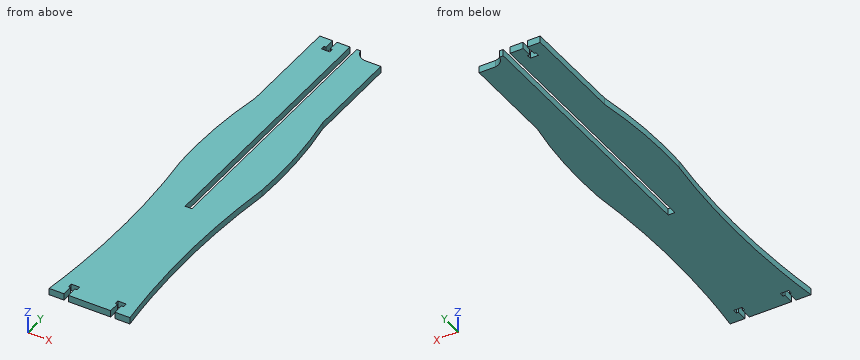
from build123d import *

# Parameters (mm, degrees)
BOSS_EXTRUDE1_DEPTH = 6.35


with BuildPart() as part:
    # Sketch2 → Boss-Extrude1 (new body)
    with BuildSketch(Plane.XY):
        with BuildLine():
            Line((-41.275, 0), (-27.223297828, 0))
            Line((-27.223297828, 0), (-27.223297828, 10.16))
            Line((-27.223297828, 10.16), (-29.128297828, 10.16))
            Line((-29.128297828, 10.16), (-29.128297828, 14.224))
            Line((-29.128297828, 14.224), (-21.254297828, 14.224))
            Line((-21.254297828, 14.224), (-21.254297828, 10.16))
            Line((-21.254297828, 10.16), (-23.159297828, 10.16))
            Line((-23.159297828, 10.16), (-23.159297828, 0))
            Line((-23.159297828, 0), (16.809297828, 0))
            Line((16.809297828, 0), (16.809297828, 10.16))
            Line((16.809297828, 10.16), (14.904297828, 10.16))
            Line((14.904297828, 10.16), (14.904297828, 14.224))
            Line((14.904297828, 14.224), (22.778297828, 14.224))
            Line((22.778297828, 14.224), (22.778297828, 10.16))
            Line((22.778297828, 10.16), (20.873297828, 10.16))
            Line((20.873297828, 10.16), (20.873297828, 0))
            Line((20.873297828, 0), (34.925, 0))
            add(Edge.make_bspline(
                [(34.925, 203.2), (22.225, 101.6), (34.925, 0)],
                knots=[0, 0, 0, 1, 1, 1], degree=2))
            add(Edge.make_bspline(
                [(28.665162854, 307.273451332), (37.499078487, 256.223776594), (34.925, 203.2)],
                knots=[0.49744374, 0.49744374, 0.49744374, 1, 1, 1], degree=2))
            Line((28.665162854, 307.273451332), (28.583690525, 396.845491603))
            Line((28.583690525, 396.845491603), (13.109843668, 396.845491603))
            ThreePointArc((13.109843668, 396.845491603), (6.812169641, 400.09411622), (3.579509775, 406.4))
            Line((3.579509775, 406.4), (0, 406.4))
            Line((0, 406.4), (0, 152.4))
            Line((0, 152.4), (-6.35, 152.4))
            Line((-6.35, 152.4), (-6.35, 406.4))
            Line((-6.35, 406.4), (-18.7325, 406.4))
            Line((-18.7325, 406.4), (-18.7325, 396.24))
            Line((-18.7325, 396.24), (-16.8275, 396.24))
            Line((-16.8275, 396.24), (-16.8275, 392.176))
            Line((-16.8275, 392.176), (-20.7645, 392.176))
            Line((-20.7645, 392.176), (-24.7015, 392.176))
            Line((-24.7015, 392.176), (-24.7015, 396.24))
            Line((-24.7015, 396.24), (-22.7965, 396.24))
            Line((-22.7965, 396.24), (-22.7965, 406.4))
            Line((-22.7965, 406.4), (-34.925, 406.4))
            Line((-34.925, 406.4), (-35.015162854, 307.273451332))
            add(Edge.make_bspline(
                [(-35.015162854, 307.273451332), (-43.849078487, 256.223776594), (-41.275, 203.2)],
                knots=[0.49744374, 0.49744374, 0.49744374, 1, 1, 1], degree=2))
            add(Edge.make_bspline(
                [(-41.275, 203.2), (-28.575, 101.6), (-41.275, 0)],
                knots=[0, 0, 0, 1, 1, 1], degree=2))
        make_face()
    extrude(amount=BOSS_EXTRUDE1_DEPTH)


solid = part.part
Read the model definition and answer for the solid it produces. Units are mm, in the model's axes. Round coordinates to 2 decimals unless told otherwise and drop trailing zeros. Order: outer loops, then holes, each group sorted by start corner. A loop starts at its lowest first (then second) coordinate and runs counter-clockwise, first axis right, second up. Notation, with made-up numbers: (-34, -39.75) - (13, -39.75) arc R13 cw to (13, -33.75) - close; hole circle Ø2 at (68.25, 15). An arc over 180 degrees is marked (long way). Use one line per item in the form item = value. Start each with the question number.
(1) Find the intervals of material crossed by line 1 along X through (y, z) = (202.5, 4.5); line 2 along Y through (x, z) = (-24, 5.5); line 3 along Y through (x, z) = (-0.5, 2.5), in increasing order. Write a range as from..to.
(2) Flat-ended cylindrical pins translate along their axes: pin 1 Ø2 at (x, z) = (22, 4.5) entering from +Y; pin 2 Ø1.9 at (x, z) = (-25, 3.5) entering from -Y; pin 3 Ø3.5 at (y, z) = (12.5, 3) entering from +X. Find the tip coordinate at first contact, or state that the pin passes through.
(3) The part is cut by section A-A (y = 319). Give the vertices of the cut face in (x, z), then the cut area to 3 significant figures.
Checked values:
q1.line_1 = -41.19..-6.35, 0..34.84
q1.line_2 = 14.22..392.18, 396.24..406.4
q1.line_3 = 0..152.4
q2.pin_1 = 396.85
q2.pin_2 = 14.22
q2.pin_3 = 33.65
q3.outline = (-35, 0) - (-6.35, 0) - (-6.35, 6.35) - (-35, 6.35) - close; (0, 0) - (28.65, 0) - (28.65, 6.35) - (0, 6.35) - close
q3.area = 364 mm^2
